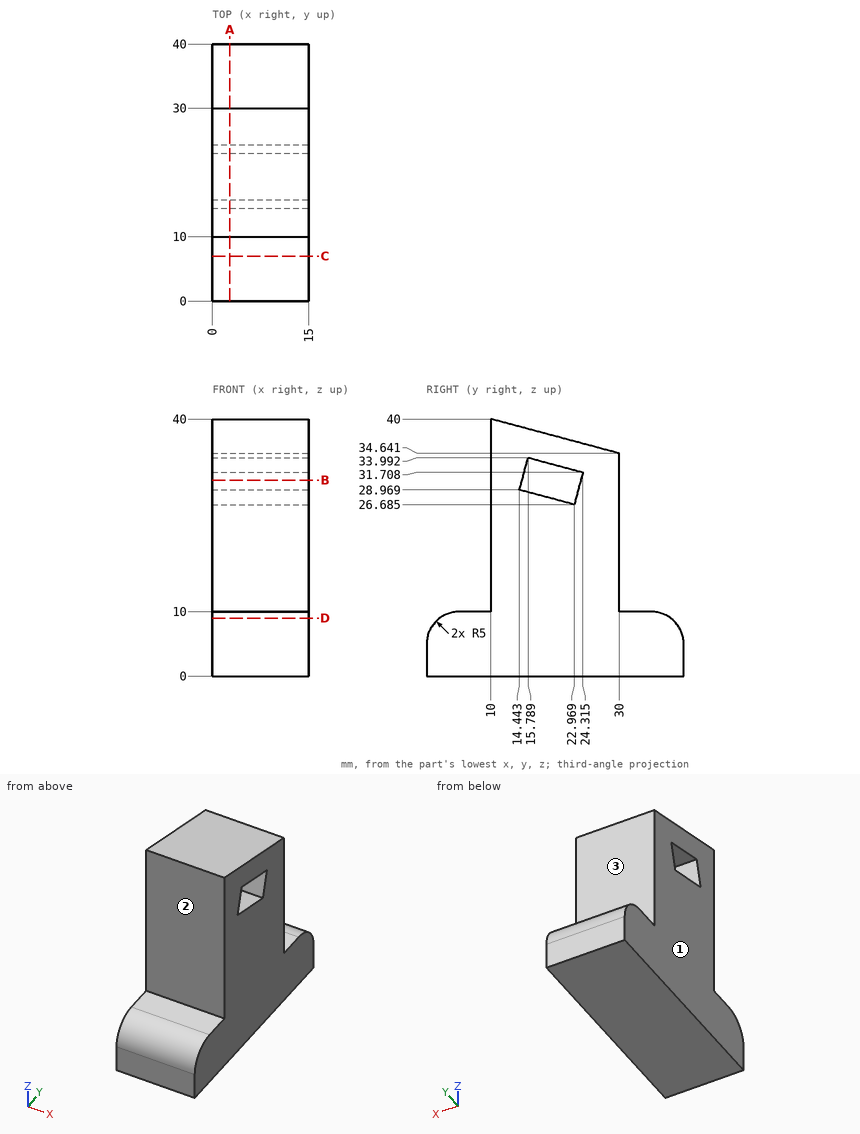
Here's the drawing with two shaded views (mm, measured from the low corner). I have some questions. A direction names the side the tool comes from. Give positions to 0.01 mm unless a question says otherwise; leave off trailing zeros. Order: outer loops, then holes, each group sorted by start corner. A loop starts at its lowest first (then second) coordinate and runs counter-clockwise, first axis right, second up. Notation, with made-up numbers: (50, 11.5) - (84, 11.5) arc R28 ccw to (84, 30.5) - close; hole circle Ø10 at (-10.75, -3.75). An arc over 180 degrees is marked (long way). Use a Markdown table: item, result. Add a question column.
Q1. On a 3-axis mill with a long thin cutter (end or side, diameter ignored), from which of +Z, -Z, +X, -X, +Y, -Y can I reach the whole of each face in a straight line? I mean the marked faces 1, 2 and 3. Say none if no direction works.
Q2. If we section it at A-A on x = 2.75: Write out the boundary of the cut face in (y, z) (1 decimal).
Q3. If we section it at B-B on z = 30.5: Write out the boundary of the cut face in (x, y), plus the area to 3 significant figures.
Q4. Please list where these lines run through material, in increasing order: line 1 along Z through (x, y) = (3.75, 34.5); line 2 along Y through (x, z) = (3.25, 29); line 3 along Z through (x, y) = (2, 21) (1 decimal).
Q5. If we section it at D-D on z = 9: Write out the boundary of the cut face in (x, y), plus the area to 3 significant figures.
Q6. If we section it at C-C on y = 7: Write out the boundary of the cut face in (x, z).
Q7. I'm going to push flat-ended pins straight in: pin 1 (1 mm diameter, centred on x = 5.5, z = 6, fed in from -Y) (1 decimal); pin 2 (4 mm diameter, centred on x = 6, y = 6.5, fed in from +Z); pin 3 (4 mm diameter, centred on x = 13.5, y = 22.5, fed in from +Z). Where does each tip first touch, or does it pass through?
Answers follow:
| question | item | result |
|---|---|---|
| 1 | face 1 | +Z, -Z, -X, +Y, -Y |
| 1 | face 2 | +Z, +X, -X, -Y |
| 1 | face 3 | +Z, +X, -X, +Y |
| 2 | outline | (0, 0) - (40, 0) - (40, 5) arc R5 ccw to (35, 10) - (30, 10) - (30, 34.6) - (10, 40) - (10, 10) - (5, 10) arc R5 ccw to (0, 5) - close; hole (14.4, 29) - (23, 26.7) - (24.3, 31.7) - (15.8, 34) - close |
| 3 | outline | (0, 10) - (15, 10) - (15, 14.85) - (0, 14.85) - close; (0, 23.99) - (15, 23.99) - (15, 30) - (0, 30) - close |
| 3 | area | 163 mm^2 |
| 4 | line 1 | z = 0 to 10 |
| 4 | line 2 | y = 10 to 14.45, 23.59 to 30 |
| 4 | line 3 | z = 0 to 27.2, 32.6 to 37.1 |
| 5 | outline | (0, 2) - (15, 2) - (15, 38) - (0, 38) - close |
| 5 | area | 540 mm^2 |
| 6 | outline | (0, 0) - (15, 0) - (15, 10) - (0, 10) - close |
| 7 | pin 1 | stops at y = 0 |
| 7 | pin 2 | stops at z = 10 |
| 7 | pin 3 | stops at z = 37.19 |
